Verification items for the finished model (mm, model axes). Face numbers are marked on the shaded views. A direction names the side the tool comes from. Give positions to 0.01 mm unless a question says otherwise; leave off trailing zeros. Write each loop counter-clockwise with the first axis right and the second up, starting at its lowest first coordinate (ties: lowest second). Pieces come first, ordered by that corner, then holes. Notation, with made-up numbers: M -13.75,41 L 20.25,41 A25 ccw 20.25,77 Z; hole C -19,55 d6. An arc over 180 degrees is marked long. Answer as a JSON object with one key per item and string values.
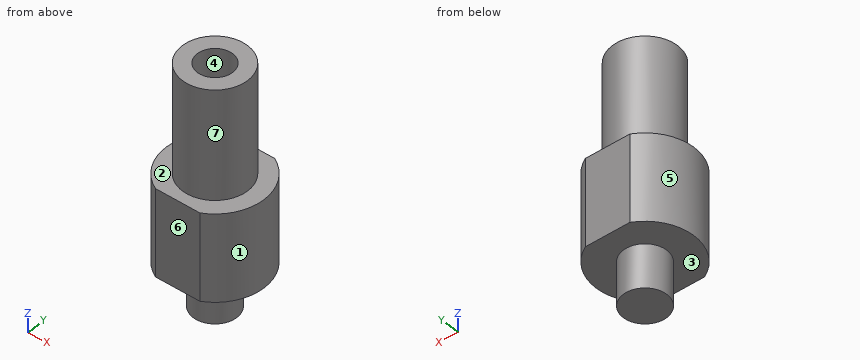
Autodesk Inventor part; units mm, degrees
ref_plane "YZ Plane" through (0, 0, 0) normal (1, 0, 0) x (0, 1, 0)
ref_plane "XZ Plane" through (0, 0, 0) normal (0, 1, 0) x (-1, 0, 0)
ref_plane "XY Plane" through (0, 0, 0) normal (0, 0, 1) x (1, 0, 0)
sketch "Skizze1" plane through (0, 0, 0) normal (0, 0, 1) x (1, 0, 0)
  line L0 (-6.3, 0) -> (6.3, 0)
  line L1 (0, -6.3) -> (0, 6.3)
  circle A0 centre (0, 0) radius 4.5
  dimension "d0" = 9
extrude "Extrusion1" add sketch "Skizze1" along normal blind 8
sketch "Skizze2" plane through (0, 0, 0) normal (0, 0, -1) x (-1, 0, 0)
  circle A0 centre (0, 0) radius 4.5
  circle A1 centre (0, 0) radius 2
  dimension "d3" = 4
extrude "Extrusion2" add sketch "Skizze2" along normal blind 4 contours A1
thread "Gewinde1"
sketch "Skizze3" plane through (0, 0, 8) normal (0, 0, 1) x (1, 0, 0)
  circle A0 centre (0, 0) radius 3
  dimension "d8" = 6
extrude "Extrusion3" add sketch "Skizze3" along normal blind 10
sketch "Skizze4" plane through (0, 0, 8) normal (0, 0, 1) x (1, 0, 0)
  circle A0 centre (0, 0) radius 3
  circle A1 centre (0, 0) radius 4.5
  line L0 (-16.8, 0) -> (16.8, 0)
  line L1 (0, -6.3) -> (0, 6.3)
  line L2 (12, 4) -> (-12, 4)
  line L3 (-12, 4) -> (-12, -4)
  line L4 (-12, -4) -> (12, -4)
  line L5 (12, -4) -> (12, 4)
  line L6 (12, 4) -> (-12, -4) construction
  line L7 (-12, 4) -> (12, -4) construction
  point P0 (-2.0616, 4)
  point P1 (2.0616, 4)
  point P2 (-2.0616, -4)
  point P3 (2.0616, -4)
  dimension "d11" = 8
extrude "Extrusion4" cut sketch "Skizze4" against normal blind 10 contours L2 A1 L1 | L1 A1 L2 | L4 A1 L1 | L1 A1 L4
sketch "Skizze5" plane through (0, 0, 18) normal (0, 0, 1) x (1, 0, 0)
  circle A0 centre (0, 0) radius 2
hole "Bohrung1" at (0, 0, 18) direction (0, 0, -1) diameter 3.242 depth 11.8 tip angle 118
properties part number "24_0497_0022"
1) Section check D-D on z = 1.25. Record the boundary of the cut face in (x, y), and give its area (3 significant figures).
Completed:
{"outline": "M -2.06,-4 L 2.06,-4 A4.5 ccw 2.06,4 L -2.06,4 A4.5 ccw Z", "area": "60.8 mm2"}
2) Go/stop test with flat-tipped pins: pin 1 (3 mm diameter, centred on y = 3, z = 5, fed in from -X); pin 2 (1.5 mm diameter, centred on x = -3.5, y = 3, fed in from -Z); pin 3 (5 mm diameter, centred on x = -0.5, z = 12, fed in from +Y). Record where each tip stops, or that it passes through.
Completed:
{"pin 1": "stops at x = -4.24", "pin 2": "stops at z = 0", "pin 3": "stops at y = 3"}
3) Access from +Z, -Z, +X, -X, +Y, -Y to the whole of each face (thin tool, end or side, straight path). Record for the marked faces 1, 2 and 3.
Completed:
{"face 1": "+Z, -Z, +X", "face 2": "+Z", "face 3": "-Z"}
4) Section check B-B on y = 2.5. Record the boundary of the cut face in (x, z), and give its area (3 significant figures).
Completed:
{"outline": "M -3.74,0 L 3.74,0 L 3.74,8 L 1.66,8 L 1.66,18 L -1.66,18 L -1.66,8 L -3.74,8 Z", "area": "93.0 mm2"}
5) Section check A-A on z = 14.75. Record the boundary of the cut face in (x, y).
Completed:
{"outline": "C 0,0 d6; hole C 0,0 d3.24"}
6) Release check for a two-part mould opening along X. For the marked faces 4, 5, 6 and 7 record: pulls with the +X half, pulls with the -X half, needs draft (parallel to the pull), parting line crosses it, or undercut.
Completed:
{"face 4": "undercut", "face 5": "pulls with the -X half", "face 6": "needs draft", "face 7": "parting line crosses it"}
7) Thickness scan on L1, parallel to Y at x = 0, z = 14.5; L2, parallel to Z at x = -1.5, y = -3.5; L3, parallel to Z at x = 0, y = 2.25. Record the ranges inside material, lowest first.
Completed:
{"L1": "y = -3 to -1.62, 1.62 to 3", "L2": "z = 0 to 8", "L3": "z = 0 to 18"}
